The listing builds one solid part. Answer for the finished solid, in the listing's coordinates (mm). A direction names the side the tool comes from. Give positions to 0.01 mm unless a question says otherwise; leave off trailing zeros. Loops run counter-clockwise (first coordinate to the right, second up) from the corner with the lowest first, then second, coordinate; pieces in that order, holes last. Notation, with made-up numbers: M 88.25,-6 L 102.25,-6 A21 ccw 102.25,15 Z; hole C 46.5,17.5 d2. An arc over 180 degrees is marked long. One line per item, written item: value. Start each with the question number.
Q1. The mould has two halves that part along Y. Classify faces 1 (the flat face through (0, -9.56, 9)), 2 (the cylindrical face through (-14.985, 0.66, 0.986)), 3 (the flat face through (0, 10, 17)): +Y half, -Y half, draft (parallel to the pull), parting line (faces both ways), or undercut.
Q2. Flat-ended cylindrical pins translate along their axes: pin 1 (10 mm diameter, centred on x = 9.5, z = 3, fed in from +Y); pin 2 (1.1 mm diameter, centred on y = -10, z = 9.5, fed in from -X); pin 3 (8 mm diameter, centred on x = 3.5, y = -9, fed in from +Z); pin 4 (10 mm diameter, centred on x = 9, y = -1, fed in from +Z). Find the tip coordinate at first contact, or state that the pin passes through.
Q3. For faces 4 (the cylindrical face through (-0.64, 6.85, 9.4)), 5 (the flat face through (-2.041, -11, 9)), 6 (the flat face through (0, -11.699, 9)), determine the directions among +Z, -Z, +X, -X, +Y, -Y from which every point of the face is accessible in a straight line to the end or side of a thin tool.
Q4. Consider L1, parallel to Z at x = -5, y = 9.75; L2, parallel to X at y = -11.5, z = 3; L3, parallel to Y at x = 2, z = 11.5. Determine where each line is inside the solid, lowest interval first.
Q5. A cutting plane is placed at D-D, the plane y = 0. Determine the outline of the cut face in (x, z).
Q6. A cutting plane is placed at B-B, the plane y = 12. Determine the outline of the cut face in (x, z).
Q7. A cutting plane is placed at A-A, the plane x = 0. Determine the outline of the cut face in (y, z).
Q8. A cutting plane is placed at C-C, the plane z = 10.25. Determine the outline of the cut face in (x, y).
from build123d import *

# Parameters (mm, degrees)
F0_R     = 15
F1_DEPTH = 2
F2_R     = 2.9516544706
F2_W     = 4.0816161782
F2_H     = 2.1391976625
F3_DEPTH = 15


# Not quite as in the source:
# - a feature names something its author has since deleted; it is built from what else it names


with BuildPart() as f1:
    # F0 (on Top) → F1 (new body)
    with BuildSketch(Plane.XY):
        Circle(F0_R)
    extrude(amount=F1_DEPTH)

    # F2 (on face) → F3 (join)
    with BuildSketch(Plane.XY.offset(2)):
        with Locations((0, 9.7299581394)):
            Circle(F2_R)
        with Locations((0, -10.6295719743)):
            Rectangle(F2_W, F2_H)
    extrude(amount=F3_DEPTH)


solid = f1.part
Answer block:
1. face 1: undercut
1. face 2: parting line
1. face 3: draft
2. pin 1: y = 14.28
2. pin 2: x = -2.04
2. pin 3: z = 17
2. pin 4: z = 2
3. face 4: +Z
3. face 5: +Z, -X, -Y
3. face 6: +Z, +X, -X, -Y
4. L1: 0 to 2
4. L2: -2.04 to 2.04
4. L3: -11.7 to -9.56, 7.56 to 11.9
5. outline: M -15,0 L 15,0 L 15,2 L -15,2 Z
6. outline: M -9,0 L 9,0 L 9,2 L 1.89,2 L 1.89,17 L -1.89,17 L -1.89,2 L -9,2 Z
7. outline: M -15,0 L 15,0 L 15,2 L 12.68,2 L 12.68,17 L 6.78,17 L 6.78,2 L -9.56,2 L -9.56,17 L -11.7,17 L -11.7,2 L -15,2 Z
8. outline: C 0,9.73 d5.9; M -2.04,-11.7 L 2.04,-11.7 L 2.04,-9.56 L -2.04,-9.56 Z
